Could you check a few things on this model? Use its own coordinates, in mm. Face numbers are marked on the shaded views. A direction names the side the tool comes from. Give positions to 0.01 mm unless a question says otherwise; leave off trailing zeros. Write each loop counter-clockwise with the first axis right and the second up, starting at its lowest first coordinate (ties: lowest second). Pieces come first, ordered by that corner, then holes. Notation, with made-up numbers: M 39.5,-16.75 L 95.5,-16.75 A25 cw 95.5,1.25 Z; hole C -16.75,-7.5 d10. An arc over 180 degrees is marked long. Use one line per item in the form item = value.
Autodesk Inventor part; units mm, degrees
ref_plane "Work Plane2" through (0, 18, 0) normal (0, 1, 0) x (1, 0, 0)
ref_plane "Work Plane3" through (50, 0, -69) normal (0, 0, -1) x (-1, 0, 0)
ref_plane "Work Plane4" through (0, 16.5, 0) normal (0, 1, 0) x (1, 0, 0)
sketch "Sketch1" plane through (0, 0, 0) normal (0, 1, 0) x (-1, 0, 0)
  line L0 (-50, 75) -> (50, 75)
  line L1 (50, 75) -> (50, -75)
  line L2 (50, -75) -> (-50, -75)
  line L3 (-50, -75) -> (-50, 75)
  line L4 (-50, 75) -> (50, -75) construction
  line L5 (50, 75) -> (-50, -75) construction
  point P0 (0, 0)
  dimension "d0" = 100
  dimension "d1" = 150
extrude "Extrusion1" add sketch "Sketch1" along normal blind 8
sketch "Sketch3" plane through (0, 8, 0) normal (0, 1, 0) x (1, 0, 0)
  line L0 (-50, -75) -> (50, -75)
  line L1 (50, -75) -> (50, 75)
  line L2 (50, 75) -> (-50, 75)
  line L3 (-50, 75) -> (-50, -75)
  line L4 (45, 75) -> (45, -70)
  line L5 (-50, -75) -> (50, -75)
  line L6 (50, -75) -> (50, 75)
  line L7 (0, 0) -> (0, -83) construction
  line L8 (-45, 75) -> (-45, -70)
  line L9 (45, -70) -> (-45, -70)
  dimension "d4" = 5
  dimension "d5" = 5
extrude "Extrusion2" add sketch "Sketch3" along normal blind 18 contours L3 L2 L8 L9 L4 L1 L0
sketch "Sketch4" plane through (50, 0, -75) normal (0, 0, -1) x (-1, 0, 0)
  line L0 (100, 0) -> (0, 0)
  line L1 (100, 0) -> (100, 26)
  line L2 (95, 26) -> (100, 26)
  line L3 (95, 8) -> (95, 26)
  line L4 (5, 8) -> (95, 8)
  line L5 (5, 8) -> (5, 26)
  line L6 (0, 26) -> (5, 26)
  line L7 (0, 0) -> (0, 26)
  line L8 (95, 8) -> (5, 8)
  line L9 (5, 8) -> (5, 0)
  line L10 (95, 8) -> (95, 0)
  line L11 (0, 0) -> (100, 0)
  line L12 (0, 0) -> (0, 26)
  line L13 (5, 3) -> (95, 3)
  line L14 (5, 8) -> (95, 8)
  line L15 (5, 6) -> (95, 6)
  line L16 (5, 8) -> (0, 8)
  line L17 (100, 0) -> (0, 0)
  point P0 (50, 0)
  dimension "d8" = 3
  dimension "d9" = 3
extrude "Extrusion3" add sketch "Sketch4" along normal blind 20 contours L0 L10 L3 L2 L1 | L0 L9 L13 L10 | L15 L9 L4 L10 | L7 L6 L5 L16
sketch "Sketch6" plane through (50, 0, 75) normal (1, 0, 0) x (0, 0, -1)
  line L0 (150, 0) -> (150, 8)
  line L1 (170, 26) -> (170, 8)
  line L2 (0, 0) -> (0, 26)
  line L3 (150, 8) -> (170, 8)
  line L4 (170, 26) -> (170, 8)
  line L5 (170, 11.2) -> (163, 9.7)
  line L6 (163, 9.7) -> (163, 15.7)
  line L7 (163, 15.7) -> (170, 14.2)
  line L8 (170, 19.3) -> (163, 17.8)
  line L9 (163, 17.8) -> (163, 23.8)
  line L10 (163, 23.8) -> (170, 22.3)
  line L11 (170, 22.3) -> (170, 19.3)
  line L12 (170, 14.2) -> (170, 11.2)
  point P0 (75, 0)
  dimension "d14" = 3
  dimension "d15" = 7
  dimension "d16" = 1.5
  dimension "d17" = 1.5
  dimension "d18" = 3
  dimension "d19" = 1.5
  dimension "d20" = 1.5
  dimension "d21" = 5.1
  dimension "d22" = 7
  dimension "d36" = 1.7
extrude "Extrusion4" cut sketch "Sketch6" against normal through all
fillet "Fillet1" radius 2 11 edges at (50, 0, 0) (50, 26, -10) (50, 13, 75) (0, 26, 75) (0, 0, 75) (-50, 26, -10) (-50, 13, 75) (-50, 0, -10) (45, 26, -12.5) (-45, 26, -12.5) (0, 26, 70)
sketch "Sketch11" plane through (-50, 9.7, -88) normal (-1, 0, 0) x (0, 0, 1)
  line L0 (9, 17.5) -> (0, 19.5)
  line L1 (0, 19.5) -> (0, 11.5)
  line L2 (0, 11.5) -> (9, 14)
  line L3 (9, 17.5) -> (9, 14)
  line L4 (9, 6) -> (0, 8.5)
  line L5 (0, 0) -> (9, 2.5)
  line L6 (0, 6) -> (0, 0)
  line L7 (9, 6) -> (9, 2.5)
  point P0 (88, -9.7)
sketch "Sketch12" plane through (-50, 2, 73) normal (-1, 0, 0) x (0, 0, 1)
  line L0 (-168, 28) -> (-168, 20)
  line L1 (-159, 26) -> (-168, 28)
  line L2 (-159, 26) -> (-159, 22.5)
  line L3 (-168, 20) -> (-159, 22.5)
  line L4 (-168, 17) -> (-168, 8.5)
  line L5 (-159, 14.5) -> (-168, 17)
  line L6 (-159, 14.5) -> (-159, 11)
  line L7 (-168, 8.5) -> (-159, 11)
  line L8 (-168, 0) -> (-168, 22)
  line L9 (-161, 19.2) -> (-161, 27.2)
  line L10 (-161, 27.2) -> (-168, 27.2)
  line L11 (-168, 22) -> (-168, 6)
  line L12 (-159, 17) -> (-168, 17)
  point P0 (-73, -2)
sketch "Sketch15" plane through (45, 6, -75) normal (1, 0, 0) x (0, 0, -1)
  line L0 (0, 0) -> (0, 2)
  line L1 (0, 0) -> (20, 0)
  line L2 (20, 2) -> (20, 0)
  line L3 (0, 2) -> (20, 2)
  point P0 (-75, -6)
extrude "Extrusion8" add sketch "Sketch15" along normal blind 2.5
sketch "Sketch16" plane through (0, 8, 0) normal (0, 1, 0) x (1, 0, 0)
  line L0 (-45, -35) -> (-37, -35)
  line L1 (-37, -35) -> (-37, -15)
  line L2 (-37, -15) -> (-45, -15)
  line L3 (-45, -15) -> (-45, -35)
  line L4 (45, -70) -> (-45, -70)
  line L5 (-45, -70) -> (-45, 95)
  line L6 (32, -70) -> (45, -70)
  line L7 (45, -70) -> (45, -45)
  line L8 (45, -45) -> (32, -45)
  line L9 (32, -45) -> (32, -70)
  line L10 (45, 95) -> (45, -70)
  point P0 (0, 0)
  dimension "d39" = 35
  dimension "d40" = 0
  dimension "d41" = 8
  dimension "d42" = 20
  dimension "d43" = 0
  dimension "d44" = 0
  dimension "d45" = 25
  dimension "d46" = 13
extrude "Extrusion9" add sketch "Sketch16" along normal blind 16
fillet "Fillet4" radius 1 8 edges at (32, 24, 57.5) (38.5, 24, 45) (32, 16, 45) (-37, 24, 25) (-37, 16, 15) (-41, 24, 35) (-41, 24, 15) (-37, 16, 35)
sketch "Sketch17" plane through (0, 24, 0) normal (0, 1, 0) x (1, 0, 0)
  circle A0 centre (-41.5, -25) radius 2.1
  line L0 (-45, -34) -> (-45, -16)
  line L1 (-38, -34) -> (-45, -34)
  circle A1 centre (39, -58) radius 2.1
  line L2 (33, -70) -> (33, -46)
  line L3 (33, -46) -> (45, -46)
  point P0 (0, 0)
  dimension "d50" = 4.2
  dimension "d51" = 3.5
  dimension "d52" = 9
  dimension "d53" = 4.2
  dimension "d54" = 6
  dimension "d55" = 12
extrude "Extrusion10" cut sketch "Sketch17" against normal blind 8
sketch "Sketch18" plane through (-45, 9.7, -88) normal (1, 0, 0) x (0, 0, -1)
  circle A0 centre (-58, 11.3) radius 2.15
  circle A1 centre (-27.2, 11.3) radius 2.15
  line L0 (0, 8.1) -> (0, 14.1)
  line L1 (-27.2, 11.3) -> (-58, 11.3)
  line L2 (7, 16.3) -> (-160, 16.3)
  line L3 (-158, -1.7) -> (-158, 14.3)
  point P0 (-88, -9.7)
  dimension "d60" = 4.3
  dimension "d61" = 4.3
  dimension "d62" = 30.8
  dimension "d64" = 5
  dimension "d67" = 100
extrude "Extrusion11" cut sketch "Sketch18" against normal through all
sketch "Sketch19" plane through (0, 24, 0) normal (0, 1, 0) x (1, 0, 0)
  circle A0 centre (-41.5, -25) radius 2.1
  line L0 (-42, -22) -> (-39.1519, -23.067)
  line L1 (-39.1519, -23.067) -> (-38.6519, -26.067)
  line L2 (-38.6519, -26.067) -> (-41, -28)
  line L3 (-41, -28) -> (-43.8481, -26.933)
  line L4 (-43.8481, -26.933) -> (-44.3481, -23.933)
  line L5 (-44.3481, -23.933) -> (-42, -22)
  point P0 (0, 0)
ref_plane "Work Plane2" through (0, 18, 0) normal (0, 1, 0) x (1, 0, 0)
ref_plane "Work Plane1" through (0, 20, 0) normal (0, 1, 0) x (1, 0, 0)
extrude "Extrusion12" cut sketch "Sketch19" against normal up to surface (2 mm away) from surface at -4
ref_plane "Work Plane3" through (50, 0, -69) normal (0, 0, -1) x (-1, 0, 0)
sketch "Sketch20" plane through (50, 0, -69) normal (0, 0, -1) x (-1, 0, 0)
  line L0 (-27, 40) -> (133, 40)
  line L1 (133, 40) -> (133, -17)
  line L2 (133, -17) -> (-27, -17)
  line L3 (-27, -17) -> (-27, 40)
  point P0 (50, 0)
extrude "Extrusion13" cut sketch "Sketch20" against normal through all
sketch "Sketch21" plane through (0, 8, 0) normal (0, 1, 0) x (1, 0, 0)
  line L0 (-25, 71) -> (-35, 71)
  line L1 (-35, 71) -> (-35, 81)
  line L2 (-35, 81) -> (-25, 81)
  line L3 (-25, 81) -> (-25, 71)
  circle A0 centre (-30, 76) radius 2.1
  line L4 (-70, 69) -> (70, 69)
  line L5 (-45, 69) -> (-45, 95)
  point P0 (0, 0)
  dimension "d76" = 4.2
  dimension "d77" = 2
  dimension "d78" = 10
  dimension "d79" = 5
  dimension "d80" = 10
  dimension "d81" = 10
  dimension "d82" = 5
extrude "Extrusion14" add sketch "Sketch21" along normal blind 10
ref_plane "Work Plane4" through (0, 16.5, 0) normal (0, 1, 0) x (1, 0, 0)
sketch "Sketch22" plane through (0, 16.5, 0) normal (0, 1, 0) x (1, 0, 0)
  line L0 (-32.0207, 72.5) -> (-34.0415, 76)
  line L1 (-34.0415, 76) -> (-32.0207, 79.5)
  line L2 (-32.0207, 79.5) -> (-27.9793, 79.5)
  line L3 (-27.9793, 79.5) -> (-25.9585, 76)
  line L4 (-25.9585, 76) -> (-27.9793, 72.5)
  line L5 (-27.9793, 72.5) -> (-32.0207, 72.5)
  point P0 (0, 0)
  point P1 (-30, 76)
  dimension "d88" = 7
extrude "Extrusion15" cut sketch "Sketch22" against normal blind 3.15
properties part number "Prova A1"
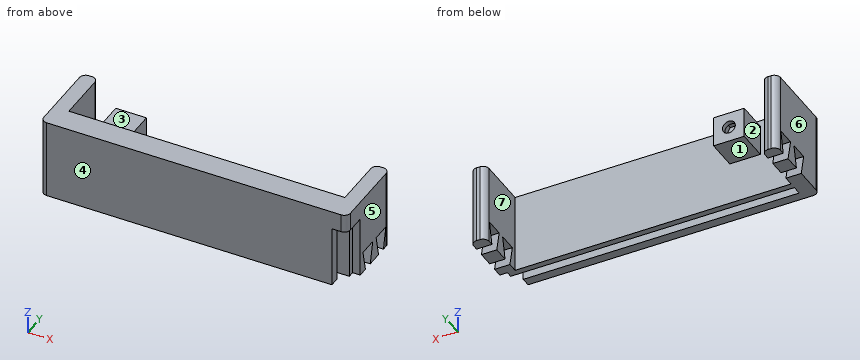
1) For pin 1 Ø1.5 at (x, y) = (39.5, 9.5) entering from -Z; pin 2 Ø5 at (x, z) = (-32, -75) entering from +Y; pin 3 Ø3 at (x, y) = (-30.5, 14.5) entering from +Z; pin 4 Ø0.9 at (x, y) = (-29.5, 15.5) entering from -Z, each with a flat end and sliding along its axis, tell me the tip position at first contact or that it passes through.
Checked values:
pin_1 = through
pin_2 = 18
pin_3 = -71
pin_4 = -81
2) I want a section at B-B, the plane y = 4. Please give me the cut outline in (x, z).
Checked values:
outline = M -50,-95 L -45,-95 L -45,-75 L 50,-75 L 50,-69 L -50,-69 Z
3) I want a section at C-C, the plane x = -8. Please give me the cut outline in (y, z).
Checked values:
outline = M 0,-95 L 3,-95 L 3,-75 L 6,-75 L 6,-95 L 8,-95 L 8,-69 L 0,-69 Z
4) I want a section at D-D, the plane z = -89.25. Count the separate pieces of the cut face and the enclosed holes in it, plus the area to 3 significant figures.
Checked values:
separate_pieces = 5
enclosed_holes = 0
area = 561 mm2
5) For the marked faces 1, 2 and 3, which set-ups out of +Z, -Z, +X, -X, +Y, -Y let a thin tool reach every point of the face, with its end or its side?
Checked values:
face_1 = -Z, +Y
face_2 = +Z, -Z, +Y
face_3 = +Z, +Y
6) Thinking about a two-plate mould opening in X: for the marked faces 4, 5, 6 and 7, which applies, released by +X, released by -X, zero draft, split by the parting line, or undercut?
Checked values:
face_4 = zero draft
face_5 = released by +X
face_6 = released by -X
face_7 = undercut
7) I want a section at A-A, the plane x = -30. Please give me the cut outline in (y, z).
Checked values:
outline = M 0,-95 L 3,-95 L 3,-75 L 6,-75 L 6,-95 L 8,-95 L 8,-81 L 18,-81 L 18,-78.1 L 16.5,-78.1 L 16.5,-79.5 L 13.35,-79.5 L 13.35,-78.1 L 8,-78.1 L 8,-73.9 L 13.35,-73.9 L 13.35,-72.5 L 16.5,-72.5 L 16.5,-73.9 L 18,-73.9 L 18,-71 L 8,-71 L 8,-69 L 0,-69 Z
8) If I drill on L1, parallel to X at y = 9.85, z = -76; L2, parallel to Z at x = -30, y = 11.25; L3, parallel to X at y = 20, z = -87, over which ranges is the centre line in solid material (lowest first)?
Checked values:
L1 = -50 to -45, -35 to -32.1, -27.9 to -25, 45 to 50
L2 = -81 to -78.1, -73.9 to -71
L3 = -50 to -45, 45 to 50
